```python
from build123d import *

# Parameters (mm, degrees)
SKETCH_1_W          = 49
SKETCH_1_H          = 39
EXTRUDE_1_DEPTH     = 4
CUT_EXTRUDE_1_DEPTH = 13
SKETCH_4_R          = 2.7
CUT_EXTRUDE_2_DEPTH = 17
SKETCH_5_R          = 2.7
SKETCH_5_R_2        = 3.2
CUT_EXTRUDE_3_DEPTH = 17


with BuildPart() as part:
    # 草图1 → 凸台-拉伸1 (new body)
    with BuildSketch(Plane.XY):
        with Locations((-31.928797257, 1.614086391)):
            Rectangle(SKETCH_1_W, SKETCH_1_H)
    extrude(amount=EXTRUDE_1_DEPTH)

    # 草图2 → 切除-拉伸1 (cut)
    with BuildSketch(Plane.XY):
        Polygon((-7.428797257, -17.885913609), (-35.428797257, -17.885913609), (5.926023005, 5.990303001), align=None)
    extrude(amount=CUT_EXTRUDE_1_DEPTH, mode=Mode.SUBTRACT)

    # 草图4 → 切除-拉伸2 (cut)
    with BuildSketch(Plane.XY):
        with Locations((-19.128797257, 2.114086391)):
            Circle(SKETCH_4_R)
    extrude(amount=CUT_EXTRUDE_2_DEPTH, mode=Mode.SUBTRACT)

    # 草图5 → 切除-拉伸3 (cut)
    with BuildSketch(Plane.XY):
        with Locations((-46.428797257, 12.114086391)):
            Circle(SKETCH_5_R)
        with Locations((-46.428797257, -7.885913609)):
            Circle(SKETCH_5_R_2)
    extrude(amount=CUT_EXTRUDE_3_DEPTH, mode=Mode.SUBTRACT)


solid = part.part
```
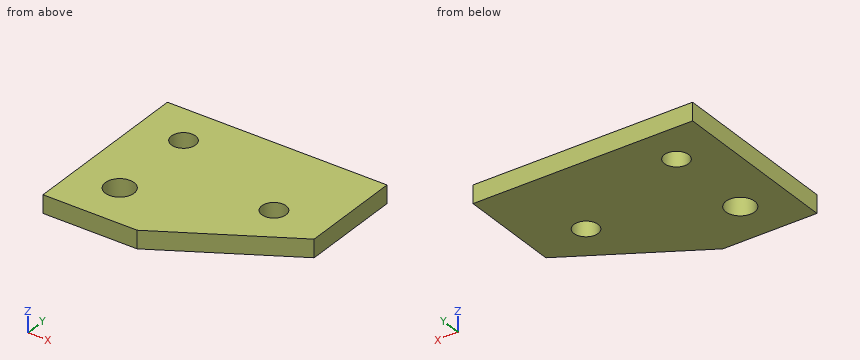
Input: part model. Units: mm. Frame: model coordinates. Coordinates: 2 decimals unless noted, no trailing zeros. Loops run counter-clockwise (first coordinate to the right, second up) from the corner with the lowest first, then second, coordinate; pieces in that order, holes last. Notation, with made-up numbers: M 23,63.5 L 53,63.5 A22 ccw 53,92.5 Z; hole C 69.5,62 d7. An arc over 180 degrees is marked long. Answer in a Markdown table with one row per item.
1. Section A-A, the plane y = -10. Output: boundary loops of the cut face in (x, z).
Response:
| item | result |
|---|---|
| outline | M -56.43,0 L -48.83,0 L -48.83,4 L -56.43,4 Z; M -44.03,0 L -21.77,0 L -21.77,4 L -44.03,4 Z |
2. Section B-B, the plane z = 1.85. Output: boundary loops of the cut face in (x, y).
Response:
| item | result |
|---|---|
| outline | M -56.43,-17.89 L -35.43,-17.89 L -7.43,-1.72 L -7.43,21.11 L -56.43,21.11 Z; hole C -46.43,-7.89 d6.4; hole C -46.43,12.11 d5.4; hole C -19.13,2.11 d5.4 |
3. Section C-C, the plane x = -17.5. Output: boundary loops of the cut face in (y, z), then the cut area to 3 significant figures.
Response:
| item | result |
|---|---|
| outline | M -7.53,0 L -0.04,0 L -0.04,4 L -7.53,4 Z; M 4.27,0 L 21.11,0 L 21.11,4 L 4.27,4 Z |
| area | 97.4 mm2 |
4. Material intervals for line 1 (Y direction, x = -46.5, z = 1.15); line 2 (Y direction, x = -48, z = 3.1); line 3 (X direction, y = 10.5, z = 3.45), sorted ascending.
Response:
| item | result |
|---|---|
| line 1 | y = -17.89 to -11.09, -4.69 to 9.42, 14.81 to 21.11 |
| line 2 | y = -17.89 to -10.67, -5.1 to 9.92, 14.31 to 21.11 |
| line 3 | x = -56.43 to -48.59, -44.26 to -7.43 |
5. Section D-D, the plane y = -3.5. Output: boundary loops of the cut face in (x, z), then the cut area to 3 significant figures.
Response:
| item | result |
|---|---|
| outline | M -56.43,0 L -10.51,0 L -10.51,4 L -56.43,4 Z |
| area | 184 mm2 |
